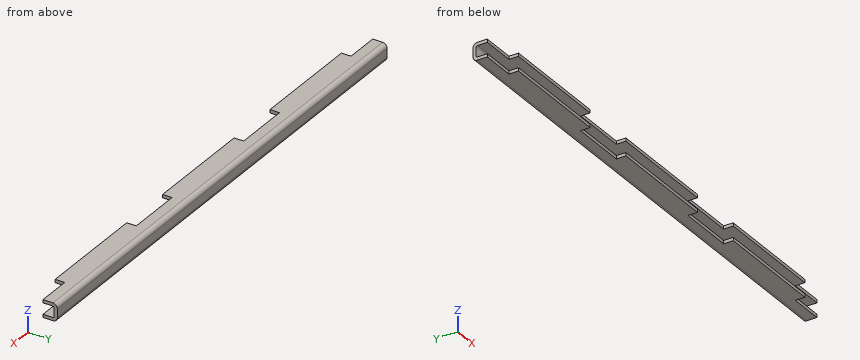
```python
from build123d import *

# Parameters (mm, degrees)
SKETCH2_W                      = 322.4
SKETCH2_H                      = 11
BASE_FLANGE1_DEPTH             = 2
EDGE_FLANGE1_STRIP_W           = 9.4732
EDGE_FLANGE1_STRIP_H           = 2
EDGE_FLANGE1_STRIP_CUT_DEPTH   = 322.4
EDGE_FLANGE1_STRIP_2_W         = 9.4732
EDGE_FLANGE1_STRIP_2_H         = 2
EDGE_FLANGE1_STRIP_CUT_2_DEPTH = 322.4
EDGE_FLANGE1_DEPTH             = 322.4
EDGE_FLANGE1_BEND_DEPTH        = 322.4
SKETCH15_W                     = 70
SKETCH15_H                     = 6
TAB1_DEPTH                     = 2


# Sheet-metal steps are written as plain solids
with BuildPart() as part:
    # Sketch2 → Base-Flange1 (new body)
    with BuildSketch(Plane(origin=(0, 0, 0), x_dir=(1, 0, 0), z_dir=(0, 1, 0))):
        Rectangle(SKETCH2_W, SKETCH2_H)
    extrude(amount=-BASE_FLANGE1_DEPTH)

    # Edge-Flange1 strip (across the edge) → Edge-Flange1 strip cut (cut)
    with BuildSketch(Plane(origin=(161.2, -2, 5.5), x_dir=(0, 0, -1), z_dir=(-1, 0, 0))):
        with Locations((-2, -1)):
            Rectangle(EDGE_FLANGE1_STRIP_W, EDGE_FLANGE1_STRIP_H)
    extrude(amount=EDGE_FLANGE1_STRIP_CUT_DEPTH, mode=Mode.SUBTRACT)

    # Edge-Flange1 strip 2 (across the edge) → Edge-Flange1 strip cut 2 (cut)
    with BuildSketch(Plane(origin=(-161.2, -2, -5.5), x_dir=(0, 0, 1), z_dir=(1, 0, 0))):
        with Locations((-2, -1)):
            Rectangle(EDGE_FLANGE1_STRIP_2_W, EDGE_FLANGE1_STRIP_2_H)
    extrude(amount=EDGE_FLANGE1_STRIP_CUT_2_DEPTH, mode=Mode.SUBTRACT)

    # Edge-Flange1 section (across the edge) → Edge-Flange1 (add)
    with BuildSketch(Plane(origin=(161.2, -2, 5.5), x_dir=(0, 0, -1), z_dir=(-1, 0, 0))):
        with BuildLine():
            Line((0, 0.7366), (0, 7))
            Line((0, 7), (2, 7))
            Line((2, 7), (2, 0.7366))
            ThreePointArc((2, 0.7366), (2.215745145, 0.215745145), (2.7366, 0))
            Line((2.7366, 0), (2.7366, -2))
            ThreePointArc((2.7366, -2), (0.801531583, -1.198468417), (0, 0.7366))
        make_face()
    extrude(amount=EDGE_FLANGE1_DEPTH)

    # Edge-Flange1 section 2 (across the edge) → Edge-Flange1 bend (add)
    with BuildSketch(Plane(origin=(-161.2, -2, -5.5), x_dir=(0, 0, 1), z_dir=(1, 0, 0))):
        with BuildLine():
            Line((0, 0.7366), (0, 7))
            Line((0, 7), (2, 7))
            Line((2, 7), (2, 0.7366))
            ThreePointArc((2, 0.7366), (2.215745145, 0.215745145), (2.7366, 0))
            Line((2.7366, 0), (2.7366, -2))
            ThreePointArc((2.7366, -2), (0.801531583, -1.198468417), (0, 0.7366))
        make_face()
    extrude(amount=EDGE_FLANGE1_BEND_DEPTH)

    # Sketch15 → Tab1 (add)
    with BuildSketch(Plane(origin=(0, 0, -5.5), x_dir=(-1, 0, 0), z_dir=(0, 0, -1))):
        with Locations((-105, -12)):
            Rectangle(SKETCH15_W, SKETCH15_H)
        with Locations((0, -12)):
            Rectangle(SKETCH15_W, SKETCH15_H)
        with Locations((105, -12)):
            Rectangle(SKETCH15_W, SKETCH15_H)
    tab1 = extrude(amount=-TAB1_DEPTH)

    # Mirror1: Tab1 across plane
    add(tab1.mirror(Plane.XY))


solid = part.part
```
The listing builds one solid part. Answer for the finished solid, in the listing's coordinates (mm). Give positions to 0.01 mm unless a question says otherwise; leave off trailing zeros. Write each loop counter-clockwise with the first axis right and the second up, starting at its lowest first coordinate (ties: lowest second). Pieces come first, ordered by that corner, then holes. Notation, with made-up numbers: (-29.5, 20.25) -> (11.5, 20.25) arc R19 ccw to (11.5, 33.25) -> close; hole circle Ø5 at (15, -11.5). An arc over 180 degrees is marked (long way). Write item = value, one per line. Start each with the question number.
1) The part is cut by section D-D, the plane x = -48.5. Determine the outline of the cut face in (y, z), and give its area (3 significant figures).
2) Each of these flat-tipped pins is pushed along its axis until it touches: pin 1 (2 mm diameter, centred on y = -12.5, z = -4.5, fed in from +X); pin 2 (2 mm diameter, centred on y = -12, z = 4.5, fed in from -X); pin 3 (2 mm diameter, centred on x = -152.5, z = 5, fed in from -Y). Where does it stop, or does it pass through?
3) The part is cut by section A-A, the plane y = -12. Determine the outline of the cut face in (x, z), and give its area (3 significant figures).
4) The part is cut by section B-B, the plane x = -8. Determine the outline of the cut face in (y, z), and give its area (3 significant figures).
5) Straight lines are drawn through the part: line 1 along Z through (x, y) = (-9, -5.75); line 2 along X through (y, z) = (-10, 4.5); line 3 along Y through (x, z) = (-1, 1). For each, find the intervals that lie inside material, in ascending order.
6) The part is cut by section C-C, the plane z = 0.75. Determine the outline of the cut face in (x, y).
Solutions:
q1.outline = (-9, -5.5) -> (-2.74, -5.5) arc R2.74 ccw to (0, -2.76) -> (0, 2.76) arc R2.74 ccw to (-2.74, 5.5) -> (-9, 5.5) -> (-9, 3.5) -> (-2.74, 3.5) arc R0.74 cw to (-2, 2.76) -> (-2, -2.76) arc R0.74 cw to (-2.74, -3.5) -> (-9, -3.5) -> close
q1.area = 47.0 mm²
q2.pin_1 = 140
q2.pin_2 = -140
q2.pin_3 = -9
q3.outline = (-140, -5.5) -> (-70, -5.5) -> (-70, -3.5) -> (-140, -3.5) -> close; (-140, 3.5) -> (-70, 3.5) -> (-70, 5.5) -> (-140, 5.5) -> close; (-35, -5.5) -> (35, -5.5) -> (35, -3.5) -> (-35, -3.5) -> close; (-35, 3.5) -> (35, 3.5) -> (35, 5.5) -> (-35, 5.5) -> close; (70, -5.5) -> (140, -5.5) -> (140, -3.5) -> (70, -3.5) -> close; (70, 3.5) -> (140, 3.5) -> (140, 5.5) -> (70, 5.5) -> close
q3.area = 840 mm²
q4.outline = (-15, -5.5) -> (-2.74, -5.5) arc R2.74 ccw to (0, -2.76) -> (0, 2.76) arc R2.74 ccw to (-2.74, 5.5) -> (-15, 5.5) -> (-15, 3.5) -> (-2.74, 3.5) arc R0.74 cw to (-2, 2.76) -> (-2, -2.76) arc R0.74 cw to (-2.74, -3.5) -> (-15, -3.5) -> close
q4.area = 71.0 mm²
q5.line_1 = -5.5 to -3.5, 3.5 to 5.5
q5.line_2 = -140 to -70, -35 to 35, 70 to 140
q5.line_3 = -2 to 0
q6.outline = (-161.2, -2) -> (161.2, -2) -> (161.2, 0) -> (-161.2, 0) -> close
